from build123d import *

# Parameters (mm, degrees)
BOSS_EXTRUDE1_DEPTH = 155
SKETCH2_W           = 6
SKETCH2_H           = 36
BOSS_EXTRUDE2_DEPTH = 2
SKETCH3_W           = 6
SKETCH3_H           = 36
BOSS_EXTRUDE3_DEPTH = 2
CUT_EXTRUDE1_REACH  = 160.584
SKETCH4_W           = 3
SKETCH4_H           = 3


with BuildPart() as part:
    # Sketch1 → Boss-Extrude1 (new body)
    with BuildSketch(Plane(origin=(0, 0, 0), x_dir=(1, 0, 0), z_dir=(0, 1, 0))):
        Polygon((0, -16), (0, 16), (-4, 16), (-4, 18), (2, 18), (2, -18), (2, -22), (0, -22), (0, -18), (-4, -18), (-4, -16), align=None)
    extrude(amount=BOSS_EXTRUDE1_DEPTH)

    # Sketch2 → Boss-Extrude2 (add)
    with BuildSketch(Plane(origin=(0, 155, 0), x_dir=(1, 0, 0), z_dir=(0, 1, 0))):
        with Locations((-1, 0)):
            Rectangle(SKETCH2_W, SKETCH2_H)
    extrude(amount=BOSS_EXTRUDE2_DEPTH)

    # Sketch3 → Boss-Extrude3 (add)
    with BuildSketch(Plane.XZ):
        with Locations((-1, 0)):
            Rectangle(SKETCH3_W, SKETCH3_H)
    extrude(amount=BOSS_EXTRUDE3_DEPTH)

    # Sketch4 → Cut-Extrude1 (cut, up to next)
    with BuildSketch(Plane(origin=(0, 0, 0), x_dir=(1, 0, 0), z_dir=(0, 1, 0)), mode=Mode.PRIVATE) as cut_extrude1_sk1:
        with Locations((-1.5, -11)):
            Rectangle(SKETCH4_W, SKETCH4_H)
    cut_extrude1_tool1 = extrude(cut_extrude1_sk1.sketch, amount=-CUT_EXTRUDE1_REACH, mode=Mode.PRIVATE) & part.part
    # Sketch4 → Cut-Extrude1 (cut, up to next)
    with BuildSketch(Plane(origin=(0, 0, 0), x_dir=(1, 0, 0), z_dir=(0, 1, 0)), mode=Mode.PRIVATE) as cut_extrude1_sk2:
        with Locations((-1.5, -3.666666667)):
            Rectangle(SKETCH4_W, SKETCH4_H)
    cut_extrude1_tool2 = extrude(cut_extrude1_sk2.sketch, amount=-CUT_EXTRUDE1_REACH, mode=Mode.PRIVATE) & part.part
    # Sketch4 → Cut-Extrude1 (cut, up to next)
    with BuildSketch(Plane(origin=(0, 0, 0), x_dir=(1, 0, 0), z_dir=(0, 1, 0)), mode=Mode.PRIVATE) as cut_extrude1_sk3:
        with Locations((-1.5, 3.666666667)):
            Rectangle(SKETCH4_W, SKETCH4_H)
    cut_extrude1_tool3 = extrude(cut_extrude1_sk3.sketch, amount=-CUT_EXTRUDE1_REACH, mode=Mode.PRIVATE) & part.part
    # Sketch4 → Cut-Extrude1 (cut, up to next)
    with BuildSketch(Plane(origin=(0, 0, 0), x_dir=(1, 0, 0), z_dir=(0, 1, 0)), mode=Mode.PRIVATE) as cut_extrude1_sk4:
        with Locations((-1.5, 11)):
            Rectangle(SKETCH4_W, SKETCH4_H)
    cut_extrude1_tool4 = extrude(cut_extrude1_sk4.sketch, amount=-CUT_EXTRUDE1_REACH, mode=Mode.PRIVATE) & part.part
    add(cut_extrude1_tool1.solids().sort_by_distance((-1.5, 0, 11))[0], mode=Mode.SUBTRACT)
    add(cut_extrude1_tool2.solids().sort_by_distance((-1.5, 0, 3.666667))[0], mode=Mode.SUBTRACT)
    add(cut_extrude1_tool3.solids().sort_by_distance((-1.5, 0, -3.666667))[0], mode=Mode.SUBTRACT)
    add(cut_extrude1_tool4.solids().sort_by_distance((-1.5, 0, -11))[0], mode=Mode.SUBTRACT)


solid = part.part
The model under review builds one solid part; all positions refer to its coordinate system, in mm. A direction names the side the tool comes from. Coordinates: 2 decimals unless noted, no trailing zeros. Write each loop counter-clockwise with the first axis right and the second up, starting at its lowest first coordinate (ties: lowest second). Pieces come first, ordered by that corner, then holes. Notation, with made-up numbers: (66.5, -24) -> (83.5, -24) arc R32 cw to (83.5, 11) -> close; hole circle Ø2 at (-34.5, 85). An arc over 180 degrees is marked (long way). Answer in a Markdown table with one row per item.
1. We need section A-A, the plane x = -1.5. State the section outline as (y, z) points, and give its area (3 significant figures).
Answers below:
| item | result |
|---|---|
| outline | (-2, -18) -> (157, -18) -> (157, 18) -> (-2, 18) -> (-2, 12.5) -> (0, 12.5) -> (0, 16) -> (155, 16) -> (155, -16) -> (0, -16) -> (0, -12.5) -> (-2, -12.5) -> close; (-2, -9.5) -> (0, -9.5) -> (0, -5.17) -> (-2, -5.17) -> close; (-2, -2.17) -> (0, -2.17) -> (0, 2.17) -> (-2, 2.17) -> close; (-2, 5.17) -> (0, 5.17) -> (0, 9.5) -> (-2, 9.5) -> close |
| area | 740 mm^2 |
2. Draft analysis for pull direction Y (two halves, no side actions). For faces 4 (the flat face through (-2, 79, 18)), 5 (the flat face through (-1, -2, 0)), 6 (the flat face through (-2, 0, 0)), state which applies: +Y half, -Y half, draft (parallel to the pull), parting line (faces both ways), or undercut.
Answers below:
| item | result |
|---|---|
| face 4 | draft |
| face 5 | -Y half |
| face 6 | undercut |
3. We need section C-C, the plane z = 14.5. State the section outline as (x, y) points.
Answers below:
| item | result |
|---|---|
| outline | (-4, -2) -> (2, -2) -> (2, 157) -> (-4, 157) -> (-4, 155) -> (0, 155) -> (0, 0) -> (-4, 0) -> close |
4. We need section B-B, the plane y = 14.5. State the section outline as (x, z) points, and give its area (3 significant figures).
Answers below:
| item | result |
|---|---|
| outline | (-4, -18) -> (2, -18) -> (2, 22) -> (0, 22) -> (0, 18) -> (-4, 18) -> (-4, 16) -> (0, 16) -> (0, -16) -> (-4, -16) -> close |
| area | 96.0 mm^2 |
5. Clearance check with a flat-ended pin moving along its axis: pin 1 Ø1 at (x, y) = (-1, -1.5) entering from +Z. State where the tip first meets the part, or that it passes through.
Answers below:
| item | result |
|---|---|
| pin 1 | stops at z = 18 |
6. Wall thickness on probe 1 along Y at (x, z) = (-0.35, -0.5); probe 2 along Z at (x, y) = (-2.6, 126.5); probe 3 along X at (y, z) = (124.5, 10.5): over which ranges is each line inside the solid? List them lowest first. Write a range as [from, to].
Answers below:
| item | result |
|---|---|
| probe 1 | y = [-2, 0], [155, 157] |
| probe 2 | z = [-18, -16], [16, 18] |
| probe 3 | x = [0, 2] |
7. For faces 1 (the flat face through (2, 79, 2)), 2 (the flat face through (-2, 76, -16)), 3 (the flat face through (0, 76, 20)), list the 3-axis set-ups (+Z, -Z, +X, -X, +Y, -Y) from which the entire face can be reached by the end or side of a thin tool; tool diameter is ignored.
Answers below:
| item | result |
|---|---|
| face 1 | +Z, -Z, +X, +Y, -Y |
| face 2 | -X |
| face 3 | +Z, -X, +Y, -Y |
